from build123d import *

# Parameters (mm, degrees)
SKETCH_R     = 24.107232
SKETCH_R_2   = 1
PAD_DEPTH    = 2
SKETCH001_R  = 2.5
PAD001_DEPTH = 4
CHAMFER_SIZE = 0.5


with BuildPart() as part:
    # Sketch → Pad (new body)
    with BuildSketch(Plane.XY):
        with Locations((23.5, 39.5)):
            Circle(SKETCH_R)
        with Locations((41.497925, 47.004978)):
            Circle(SKETCH_R_2, mode=Mode.SUBTRACT)
        with Locations((8.001536, 51.334171)):
            Circle(SKETCH_R_2, mode=Mode.SUBTRACT)
        with Locations((21.000539, 20.160851)):
            Circle(SKETCH_R_2, mode=Mode.SUBTRACT)
        with Locations((23.5, 39.5)):
            Circle(SKETCH_R_2, mode=Mode.SUBTRACT)
    extrude(amount=PAD_DEPTH)

    # Sketch001 (on Face7 of Pad) → Pad001 (join)
    with BuildSketch(Plane.XY.offset(2)):
        with Locations((28.5, 34.5)):
            Circle(SKETCH001_R)
        with Locations((28.5, 54.5)):
            Circle(SKETCH001_R)
        with Locations((8.5, 44.5)):
            Circle(SKETCH001_R)
    extrude(amount=-PAD001_DEPTH)

    # Chamfer
    chamfer_edges = [part.edges().sort_by_distance(p)[0] for p in [
        (26, 34.5, -2),
        (26, 54.5, -2),
        (6, 44.5, -2),
    ]]
    chamfer(chamfer_edges, length=CHAMFER_SIZE)


solid = part.part
Read the model definition and answer for the solid it produces. Units are mm, in the model's axes. A direction names the side the tool comes from. Round coordinates to 2 decimals unless told otherwise and drop trailing zeros. Loops run counter-clockwise (first coordinate to the right, second up) from the corner with the lowest first, then second, coordinate; pieces in that order, holes last.
Q1. Determine the mould class of faces 1 (the face through (29, 40, 2)), 2 (the face through (34.6, 18.1, 1)), 3 (the face through (21.538, 21.004, 0.986)) for opening direction Y: released by +Y, released by -Y, zero draft, split by the parting line, or undercut.
Q2. Which of the six approach directions +Z, -Z, +X, -X, +Y, -Y give full straight-line access (tool end or side, diameter ignored) to faces 4 (the face through (28, 35, -2)), 5 (the face through (7.96, 42.06, -0.74))?
Q3. Each of these flat-tipped pins is pushed along its axis until it touches: pin 1 (1.2 mm diameter, centred on x = 41.5, y = 47, fed in from -Z); pin 2 (6 mm diameter, centred on x = 41.5, y = 34.5, fed in from -Z); pin 3 (2 mm diameter, centred on x = 13.5, z = 1.5, fed in from +Y). Where does it stop, or does it pass through?
Q4. Section A-A on y = 39.5 is taken. Write down the section's boundary in (x, z), and give its area (3 significant figures).
Q5. Section C-C on x = 28.5 is taken. Write down the section's boundary in (y, z).
Q6. Section B-B on z = -0.65 is taken. Write down the section's boundary in (x, y), and give its area (3 significant figures).
Q7. Section D-D on y = 34.5 is taken. Write down the section's boundary in (x, z), and give its area (3 significant figures).
Q8. Consider probe 1 along Z at (x, y) = (35, 28.5); probe 2 along Y at (x, z) = (23, 1.25); probe 3 along X at (y, z) = (47, 1.8). Determine where each line is inside the solid, lowest interval first.
Output:
1. face 1: zero draft
1. face 2: split by the parting line
1. face 3: undercut
2. face 4: -Z, +X, -X, +Y, -Y
2. face 5: -Z
3. pin 1: passes through
3. pin 2: stops at z = 0
3. pin 3: stops at y = 61.86
4. outline: (-0.61, 0) - (22.5, 0) - (22.5, 2) - (-0.61, 2) - close; (24.5, 0) - (47.61, 0) - (47.61, 2) - (24.5, 2) - close
4. area: 92.4 mm2
5. outline: (15.92, 0) - (32, 0) - (32, -1.5) - (32.5, -2) - (36.5, -2) - (37, -1.5) - (37, 0) - (52, 0) - (52, -1.5) - (52.5, -2) - (56.5, -2) - (57, -1.5) - (57, 0) - (63.08, 0) - (63.08, 2) - (15.92, 2) - close
6. outline: circle Ø5 at (8.5, 44.5); circle Ø5 at (28.5, 34.5); circle Ø5 at (28.5, 54.5)
6. area: 58.9 mm2
7. outline: (-0.08, 0) - (26, 0) - (26, -1.5) - (26.5, -2) - (30.5, -2) - (31, -1.5) - (31, 0) - (47.08, 0) - (47.08, 2) - (-0.08, 2) - close
7. area: 104 mm2
8. probe 1: z = 0 to 2
8. probe 2: y = 15.4 to 38.63, 40.37 to 63.6
8. probe 3: x = 0.59 to 40.5, 42.5 to 46.41
